from build123d import *

# Parameters (mm, degrees)
SKETCH1_R             = 3.6
BOSS_EXTRUDE1_DEPTH   = 5
CORTAR_EXTRUIR1_START = -2
CORTAR_EXTRUIR1_DEPTH = 2
CROQUIS3_W            = 33
CROQUIS3_H            = 13
CORTAR_EXTRUIR2_DEPTH = 2.2
CORTAR_EXTRUIR3_DEPTH = 3
CROQUIS6_R            = 1.5
CORTAR_EXTRUIR4_DEPTH = 3


with BuildPart() as part:
    # Sketch1 → Boss-Extrude1 (new body)
    with BuildSketch(Plane(origin=(0, 0, 0), x_dir=(-1, 0, 0), z_dir=(0, 0, -1))):
        with BuildLine():
            Line((-70, 0), (-61, 0))
            ThreePointArc((-61, 0), (-35, -3.837363086), (-9, 0))
            Line((-9, 0), (0, 0))
            ThreePointArc((0, 0), (15, -15), (0, -30))
            Line((0, -30), (-9, -30))
            ThreePointArc((-9, -30), (-35, -26.162636914), (-61, -30))
            Line((-61, -30), (-70, -30))
            ThreePointArc((-70, -30), (-85, -15), (-70, 0))
        make_face()
        with Locations(Location((0, -15, 0), (0, 0, 180))):
            Circle(SKETCH1_R, mode=Mode.SUBTRACT)
    extrude(amount=-BOSS_EXTRUDE1_DEPTH)

    # Croquis1 → Cortar-Extruir1 (cut)
    with BuildSketch(Plane.XY.offset(5).offset(CORTAR_EXTRUIR1_START)):
        with BuildLine():
            Line((14.08705036, -12.406737159), (0.258992817, -11.409328375))
            ThreePointArc((0.258992817, -11.409328375), (2.635562003, -12.547692326), (3.6, -15))
            ThreePointArc((3.6, -15), (2.635561992, -17.452307685), (0.258992787, -18.590671627))
            Line((0.258992787, -18.590671627), (14.08705036, -17.593262841))
            ThreePointArc((14.08705036, -17.593262841), (16.5, -15), (14.08705036, -12.406737159))
        make_face()
        with BuildLine():
            Line((0.258992817, -11.409328375), (-1.12381295, -11.309587495))
            ThreePointArc((-1.12381295, -11.309587495), (-5.09, -15), (-1.12381295, -18.690412505))
            Line((-1.12381295, -18.690412505), (0.258992787, -18.590671627))
            ThreePointArc((0.258992787, -18.590671627), (-3.6, -14.999999985), (0.258992817, -11.409328375))
        make_face()
    extrude(amount=CORTAR_EXTRUIR1_DEPTH, mode=Mode.SUBTRACT)

    # Croquis3 → Cortar-Extruir2 (cut)
    with BuildSketch(Plane(origin=(0, 0, 0), x_dir=(-1, 0, 0), z_dir=(0, 0, -1))):
        with Locations((-63.5, -15)):
            Rectangle(CROQUIS3_W, CROQUIS3_H)
    extrude(amount=-CORTAR_EXTRUIR2_DEPTH, mode=Mode.SUBTRACT)

    # Croquis4 → Cortar-Extruir3 (cut)
    with BuildSketch(Plane(origin=(0, 0, 2.2), x_dir=(-1, 0, 0), z_dir=(0, 0, -1))):
        with BuildLine():
            Line((-64.2, -9.746429785), (-68.724590164, -12.416276944))
            ThreePointArc((-68.724590164, -12.416276944), (-70.2, -15), (-68.724590164, -17.583723056))
            Line((-68.724590164, -17.583723056), (-64.2, -20.253570215))
            ThreePointArc((-64.2, -20.253570215), (-55, -15), (-64.2, -9.746429785))
        make_face()
    extrude(amount=-CORTAR_EXTRUIR3_DEPTH, mode=Mode.SUBTRACT)

    # Croquis6 → Cortar-Extruir4 (cut)
    with BuildSketch(Plane(origin=(0, 0, 2.2), x_dir=(-1, 0, 0), z_dir=(0, 0, -1))):
        with Locations((-50.5, -15)):
            Circle(CROQUIS6_R)
        with Locations((-76.7, -15)):
            Circle(CROQUIS6_R)
    extrude(amount=-CORTAR_EXTRUIR4_DEPTH, mode=Mode.SUBTRACT)


solid = part.part
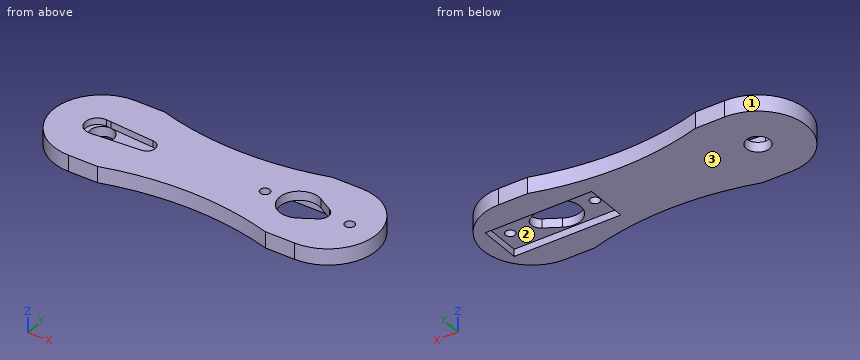
Verification items for the finished model (mm, model axes). Face numbers are marked on the shaded views. Coordinates: 2 decimals unless noted, no trailing zeros. Write each loop counter-clockwise with the first axis right and the second up, starting at its lowest first coordinate (ties: lowest second). Pieces come first, ordered by that corner, then holes. Notation, with made-up numbers: M 53,-7 L 60,-7 A12 ccw 60,7 Z; hole C 68,-30 d7. An arc over 180 degrees is marked long. One line per question, with ' | ' between items.
1) Sectioned sample at D-D on x = 74. Record the cut outline in (y, z).
Solutions:
outline: M -29.46,0 L -21.5,0 L -21.5,2.2 L -8.5,2.2 L -8.5,0 L -0.54,0 L -0.54,5 L -29.46,5 Z
2) Sectioned sample at A-A on z = 0.85. Record the cut outline in (x, y).
Solutions:
outline: M 0,-30 L 9,-30 A90 cw 61,-30 L 70,-30 A15 ccw 70,0 L 61,0 A90 cw 9,0 L 0,0 A15 ccw Z; hole C 0,-15 d7.2; hole M 47,-21.5 L 80,-21.5 L 80,-8.5 L 47,-8.5 Z
3) Release check for a two-part mould opening along Y. For the marked faces 1, 2 and 3 record: +Y half, -Y half, draft (parallel to the pull), parting line (faces both ways), or undercut.
Solutions:
face 1: parting line | face 2: undercut | face 3: draft
4) Material ranges on L1, parallel to Y at x = 61.1, z = 3.2; L2, parallel to X at y = -17, z = 0.75; L3, parallel to Y at x = 50.5, z = 3.6, recorded low to high.
Solutions:
L1: -30 to -21.1, -8.9 to 0 | L2: -14.87 to -2.99, 2.99 to 47, 80 to 84.87 | L3: -27.51 to -16.5, -13.5 to -2.49
5) Sectioned sample at C-C on x = 62.5. Record the cut outline in (y, z).
Solutions:
outline: M -30,0 L -21.5,0 L -21.5,2.2 L -20.94,2.2 L -20.94,5 L -30,5 Z; M -9.06,2.2 L -8.5,2.2 L -8.5,0 L 0,0 L 0,5 L -9.06,5 Z
6) Sectioned sample at B-B on y = -15. Record the cut outline in (x, z), then the cut area to 3 significant figures.
Solutions:
outline: M -15,0 L -3.6,0 L -3.6,3 L -5.09,3 L -5.09,5 L -15,5 Z; M 3.6,0 L 47,0 L 47,2.2 L 49,2.2 L 49,5 L 16.5,5 L 16.5,3 L 3.6,3 Z; M 52,2.2 L 55,2.2 L 55,5 L 52,5 Z; M 70.2,2.2 L 75.2,2.2 L 75.2,5 L 70.2,5 Z; M 78.2,2.2 L 80,2.2 L 80,0 L 85,0 L 85,5 L 78.2,5 Z | area: 303 mm^2
7) Depth check by flat-ended pin: pin 1 Ø0.7 at (y, z) = (-16, 1.5) entering from -X; pin 2 Ø0.7 at (x, z) = (56.5, 1.5) entering from +Y; pin 3 Ø2.5 at (x, y) = (50.5, -15) entering from +Z; pin 4 Ø1 at (x, z) = (20.5, 1) entering from -Y. Enter the tip coordinate at first touch or a pass-through.
Solutions:
pin 1: x = -14.99 | pin 2: y = -1.14 | pin 3: through | pin 4: y = -27.42
